Part model, mm, in its own coordinate system. Round coordinates to 2 decimals unless told otherwise and drop trailing zeros. Write each loop counter-clockwise with the first axis right and the second up, starting at its lowest first coordinate (ties: lowest second). Pieces come first, ordered by that corner, then holes. Notation, with made-up numbers: M 82.5,58 L 111.5,58 A9 cw 111.5,71 Z; hole C -22.5,77.5 d8. An arc over 180 degrees is marked long. Use one line per item in the form item = value. Start each with the question number.
Item 1: Flat gauge pin, fed straight in: pin 1 Ø1 at (y, z) = (95, -2.5) entering from +X. Where does the tip first touch, or does it go through?
Item 2: Cut at C-C, the plane y = 108.5. Give the cut face in (x, z) (3 decimals).
Item 3: Cut at B-B, the plane z = -2.45. Give the cut face in (x, y), then the cut area to 3 significant figures.
Item 4: Probe L1, parallel to Y at x = -190, z = -2.8; L2, parallel to X at y = 104, z = -0.2; L3, parallel to X at y = 104.75, z = -2.9. List the from-to ranges inside material, lowest first.
Item 5: Cut at D-D, the plane x = -166. Give the cut face in (y, z) (3 decimals), then the cut area to 3 significant figures.
Item 6: Mould opens along Y. For faces 1 (the face through (-215.35, 104.65, -1.57)), 2 (the face through (-190.55, 109.43, -1.57)), 3 (the face through (-190, 110, -3.175)), 4 (the face through (-164.456, 104.295, -1.565)) say: +Y half, -Y half, draft (parallel to the pull), parting line (faces both ways), or undercut.
Item 7: Cut at A-A, the plane y = 101.75. Give the cut face in (x, z) (3 decimals), then the cut area to 3 significant figures.
from build123d import *

# Parameters (mm, degrees)
SKETCH1_R           = 5
BOSS_EXTRUDE1_DEPTH = 3.175


with BuildPart() as part:
    # Sketch1 → Boss-Extrude1 (new body)
    with BuildSketch(Plane.XY):
        Polygon((-218.70690504, 117.173081746), (-211.900995552, 91.773081746), (-161.100995552, 91.773081746), (-167.90690504, 117.173081746), align=None)
        with Locations((-189.903950296, 104.473081746)):
            Circle(SKETCH1_R, mode=Mode.SUBTRACT)
    extrude(amount=-BOSS_EXTRUDE1_DEPTH)


solid = part.part
Model answer:
q1.pin_1 = -161.83
q2.outline = M -216.383,-3.175 L -192.868,-3.175 L -192.868,0 L -216.383,0 Z; M -186.94,-3.175 L -165.583,-3.175 L -165.583,0 L -186.94,0 Z
q3.outline = M -218.71,117.17 L -211.9,91.77 L -161.1,91.77 L -167.91,117.17 Z; hole C -189.9,104.47 d10
q3.area = 1,210 mm²
q4.L1 = 91.77 to 99.47, 109.47 to 117.17
q4.L2 = -215.18 to -194.88, -184.93 to -164.38
q4.L3 = -215.38 to -194.9, -184.91 to -164.58
q5.outline = M 91.773,-3.175 L 110.056,-3.175 L 110.056,0 L 91.773,0 Z
q5.area = 58.0 mm²
q6.face_1 = -Y half
q6.face_2 = undercut
q6.face_3 = draft
q6.face_4 = +Y half
q7.outline = M -214.574,-3.175 L -194.097,-3.175 L -194.097,0 L -214.574,0 Z; M -185.711,-3.175 L -163.774,-3.175 L -163.774,0 L -185.711,0 Z
q7.area = 135 mm²
